Part print with two shaded views. Sizes in mm from the minimum x, y, z corner. Round coordinates to 2 decimals unless told otherwise and drop trailing zeros. Loops run counter-clockwise (first coordinate to the right, second up) from the corner with the lowest first, then second, coordinate; pieces in that order, holes last. Notation, with made-up numbers: (82, 75.5) - (134, 75.5) arc R15 cw to (134, 104.5) - close; hole circle Ø10 at (0.5, 65). An arc over 180 degrees is marked (long way). Write each question's results on one line, items separated by ' | '. Start each with the question number.
(1) Cut at B-B, the plane x = 22.75. List the corners of the cut face in (y, z).
(2) Mould opens along Z. For the marked faces 1, 2 and 3 say: released by +Z, released by -Z, zero draft, split by the parting line, or undercut.
(3) Cut at C-C, the plane z = 18.5. List the corners of the cut face in (x, y).
(4) Cut at A-A, the plane y = 1.1. List the corners of the cut face in (x, z) (1 decimal).
(5) Drill centre lines: L1, parallel to Z at x = 7.25, y = 1.3; L2, parallel to X at y = 0.65, z = 17.75 (1 decimal); L3, parallel to Z at x = 22, y = 1.65. Where is each one in solid material? Low to high.
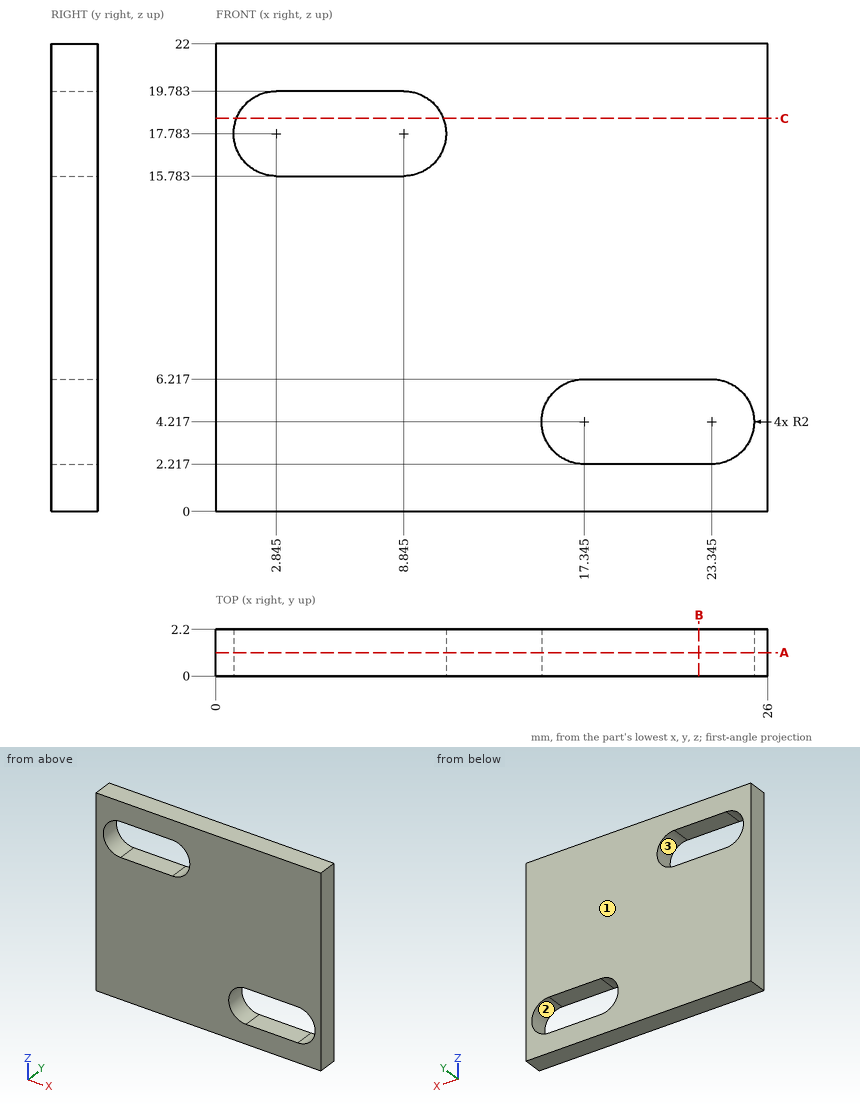
A:
1) outline: (0, 0) - (2.2, 0) - (2.2, 2.22) - (0, 2.22) - close; (0, 6.22) - (2.2, 6.22) - (2.2, 22) - (0, 22) - close
2) face 1: zero draft | face 2: undercut | face 3: undercut
3) outline: (0, 0) - (0.98, 0) - (0.98, 2.2) - (0, 2.2) - close; (10.71, 0) - (26, 0) - (26, 2.2) - (10.71, 2.2) - close
4) outline: (0, 0) - (26, 0) - (26, 22) - (0, 22) - close; hole (2.8, 15.8) - (8.8, 15.8) arc R2 ccw to (8.8, 19.8) - (2.8, 19.8) arc R2 ccw to start; hole (17.3, 2.2) - (23.3, 2.2) arc R2 ccw to (23.3, 6.2) - (17.3, 6.2) arc R2 ccw to start
5) L1: 0 to 15.78, 19.78 to 22 | L2: 0 to 0.8, 10.8 to 26 | L3: 0 to 2.22, 6.22 to 22
